from build123d import *

# Parameters (mm, degrees)
CYLINDER008_R          = 5
CYLINDER008_DEPTH      = 10
CYLINDER007_R          = 2.1
CYLINDER007_DEPTH      = 10
ARRAY001_X_COUNT       = 2
ARRAY001_X_PITCH       = 14
ARRAY001_Y_COUNT       = 2
ARRAY001_Y_PITCH       = 16
BOX006_W               = 33
BOX006_H               = 27
BOX006_DEPTH           = 3
FILLET002_R            = 3
CUT004_PITCH_ANGLE     = -90
CUT004_PLACEMENT_ANGLE = -90


with BuildPart() as motor_holder_central_hole:
    # Cylinder008 → Cylinder008 (new body)
    with BuildSketch(Plane(origin=(18, 13.5, 0), x_dir=(1, 0, 0), z_dir=(0, 0, 1))):
        Circle(CYLINDER008_R)
    extrude(amount=CYLINDER008_DEPTH)


with BuildPart() as hole_extract:
    # Cylinder007 → Cylinder007 (new body)
    with BuildSketch(Plane.XY):
        Circle(CYLINDER007_R)
    extrude(amount=CYLINDER007_DEPTH)

    # Array001 X: hole extract ×2


with BuildPart() as hole_extract_1:
    add(hole_extract.part)
    with Locations(*[(i * ARRAY001_X_PITCH, 0, 0) for i in range(1, ARRAY001_X_COUNT)]):
        add(hole_extract.part)

    # Array001 Y: hole extract ×2


with BuildPart() as hole_extract_2:
    add(hole_extract_1.part)
    with Locations(*[(0, i * ARRAY001_Y_PITCH, 0) for i in range(1, ARRAY001_Y_COUNT)]):
        add(hole_extract_1.part)


with BuildPart() as hole_extract_3:
    # Array001 placement: moved
    add(hole_extract_2.part.moved(Location((11, 5.5, 0))))

    # Fusion008: union motor holder central hole
    add(motor_holder_central_hole.part)


with BuildPart() as motor_holder_cut001:
    # Box006 → Box006 (new body)
    with BuildSketch(Plane.XY):
        with Locations((16.5, 13.5)):
            Rectangle(BOX006_W, BOX006_H)
    extrude(amount=BOX006_DEPTH)

    # Fillet002
    fillet002_edges = [motor_holder_cut001.edges().sort_by_distance(p)[0] for p in [
        (33, 0, 1.5),
        (33, 27, 1.5),
    ]]
    fillet(fillet002_edges, radius=FILLET002_R)

    # Cut004: cut hole extract
    add(hole_extract_3.part, mode=Mode.SUBTRACT)


with BuildPart() as motor_holder_cut001_1:
    # Cut004 pitch: moved
    add(motor_holder_cut001.part.rotate(Axis((0, 0, 0), (0, 1, 0)), CUT004_PITCH_ANGLE))


with BuildPart() as motor_holder_cut001_2:
    # Cut004 placement: moved
    add(motor_holder_cut001_1.part.moved(Location((-13.5, -34, 0))).rotate(Axis((-13.5, -34, 0), (0, 0, 1)), CUT004_PLACEMENT_ANGLE))


with BuildPart() as motor_holder_cut001_3:
    # Cut004001 placement: moved
    add(motor_holder_cut001_2.part.moved(Location((0, 2, 0))))


solid = motor_holder_cut001_3.part
Could you check a few things on this model? Use its own coordinates, in mm. Round coordinates to 2 decimals unless told otherwise and drop trailing zeros. Order: outer loops, then holes, each group sorted by start corner. A loop starts at its lowest first (then second) coordinate and runs counter-clockwise, first axis right, second up.
(1) Imagine slicing it at D-D (y = -31.35). Write out the boundary of the cut face in (x, z).
Response values:
outline: (-13.5, 0) - (13.5, 0) - (13.5, 30) arc R3 ccw to (10.5, 33) - (-10.5, 33) arc R3 ccw to (-13.5, 30) - close; hole circle Ø4.2 at (-8, 11); hole circle Ø4.2 at (-8, 25); hole circle Ø10 at (0, 18); hole circle Ø4.2 at (8, 11); hole circle Ø4.2 at (8, 25)
(2) Imagine slicing it at C-C (z = 18). Write out the boundary of the cut face in (x, y).
Response values:
outline: (-13.5, -32) - (-5, -32) - (-5, -29) - (-13.5, -29) - close; (5, -32) - (13.5, -32) - (13.5, -29) - (5, -29) - close
(3) I'm going to push a flat-ended pin straight in: pin 1 (4 mm diameter, centred on x = 8, z = 11, fed in from +Y). Where does the tip first touch, or does it pass through?
Response values:
pin 1: passes through
(4) Imagine slicing it at A-A (z = 11). Write out the boundary of the cut face in (x, y).
Response values:
outline: (-13.5, -32) - (-10.1, -32) - (-10.1, -29) - (-13.5, -29) - close; (-5.9, -32) - (5.9, -32) - (5.9, -29) - (-5.9, -29) - close; (10.1, -32) - (13.5, -32) - (13.5, -29) - (10.1, -29) - close
(5) Please list where these lines run through material, in increasing order: line 1 along Z through (x, y) = (8, -30.55); line 2 along X through (y, z) = (-30.1, 25); line 3 along Z through (x, y) = (-6.75, -30.9).
Response values:
line 1: z = 0 to 8.9, 13.1 to 22.9, 27.1 to 33
line 2: x = -13.5 to -10.1, -5.9 to 5.9, 10.1 to 13.5
line 3: z = 0 to 9.31, 12.69 to 23.31, 26.69 to 33
(6) Imagine slicing it at B-B (x = -8). Write out the boundary of the cut face in (y, z).
Response values:
outline: (-32, 0) - (-29, 0) - (-29, 8.9) - (-32, 8.9) - close; (-32, 13.1) - (-29, 13.1) - (-29, 22.9) - (-32, 22.9) - close; (-32, 27.1) - (-29, 27.1) - (-29, 33) - (-32, 33) - close
(7) If we mould it in two halves opening along Z, with no side actions, what happens to faces 1 (the flat face through (0.2, -32, 12.6)), 2 (the cylindrical face through (-6.23, -30.52, 26.13)), 3 (the flat face through (0, -31, 0))? For each: released by +Z, released by -Z, zero draft, split by the parting line, or undercut.
Response values:
face 1: zero draft
face 2: undercut
face 3: released by -Z
